The figure shows three views and two pictorial views of one solid part (mm, origin at its lowest corner). Answer the questions. Coordinates: 2 decimals unless noted, no trailing zeros. Loops run counter-clockwise (first coordinate to the right, second up) from the corner with the lowest first, then second, coordinate; pieces in that order, holes last. Notation, with made-up numbers: M 24,-29 L 53,-29 A19 cw 53,-21 Z; hole C 84.5,82.5 d7. An arc over 180 degrees is marked long. Answer in a Markdown table with one row per item. Add a question column.
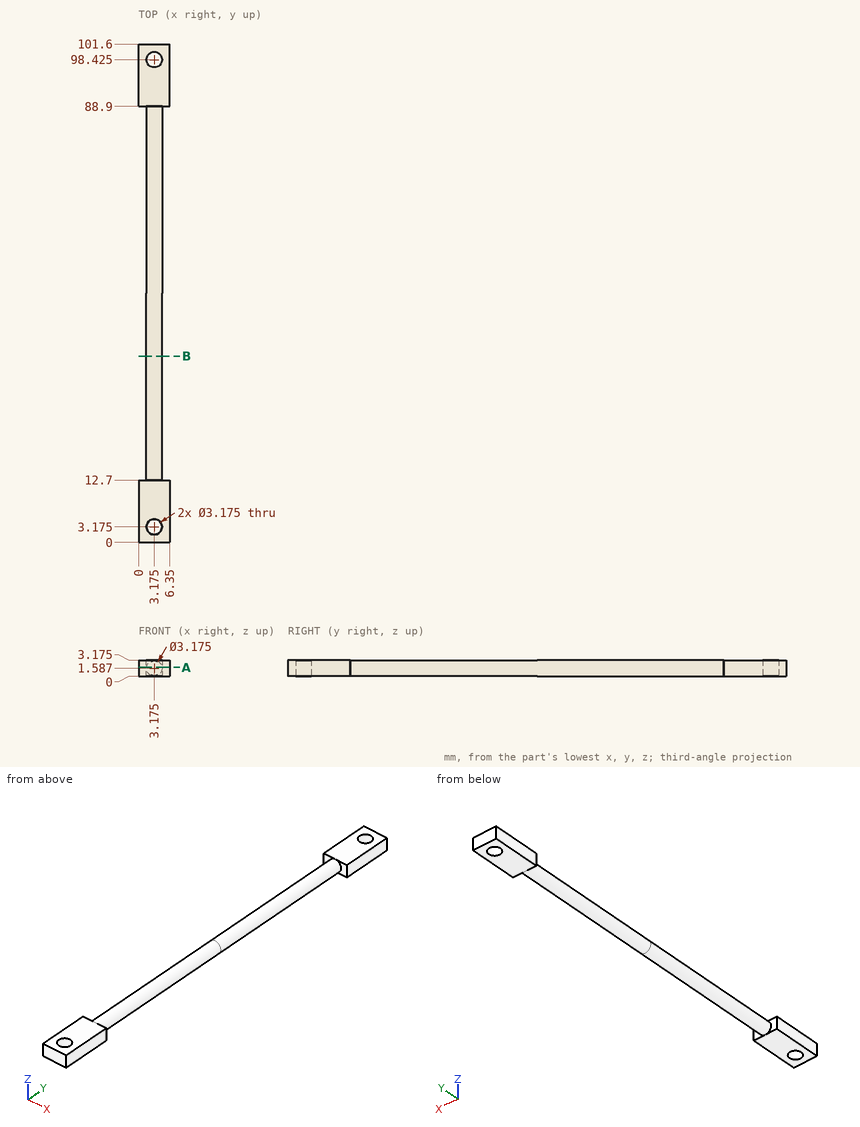
(1) Straight lines are drawn through the part: line 1 (Y direction, x = 3.25, z = 0.6); line 2 (Y direction, x = 0.75, z = 1.05); line 3 (Y direction, x = 3.75, z = 1.25) (1 decimal). For each, find the intervals that lie inside material, in ascending order.
(2) A cutting plane is placed at B-B (y = 38). Give the vertices of the cut face in (x, z) (1 decimal).
(3) Each of these flat-tipped pins is pushed along its axis until it touches: pin 1 (1.6 mm diameter, centred on x = 1, z = 2, fed in from -Y); pin 2 (1.5 mm diameter, centred on x = 2, y = 63.5, fed in from -Z). Where does it stop, or does it pass through?
(4) A cutting plane is placed at A-A (z = 1.75). State how many separate pieces and enclosed holes the cut face has, plus the area to 3 significant figures.
Solved:
| question | item | result |
|---|---|---|
| 1 | line 1 | y = 0 to 1.59, 4.76 to 96.84, 100.01 to 101.6 |
| 1 | line 2 | y = 0 to 12.7, 88.9 to 101.6 |
| 1 | line 3 | y = 0 to 1.7, 4.7 to 96.9, 99.9 to 101.6 |
| 2 | outline | C 3.2,1.6 d3.2 |
| 3 | pin 1 | stops at y = 0 |
| 3 | pin 2 | stops at z = 0.06 |
| 4 | separate pieces | 1 |
| 4 | enclosed holes | 2 |
| 4 | area | 386 mm² |
